Source: CAD feature listing. Evaluate the final solid. Frame: model axes, mm. Face numbers are marked on the shaded views. A direction names the side the tool comes from. Round coordinates to 2 decimals unless told otherwise and drop trailing zeros. Write each loop counter-clockwise with the first axis right and the second up, starting at its lowest first coordinate (ties: lowest second). Pieces come first, ordered by that corner, then holes. Notation, with made-up numbers: (87, 72.5) -> (120, 72.5) arc R19 cw to (120, 105.5) -> close; hole circle Ø5 at (-31.75, -33). An arc over 180 degrees is marked (long way). Return JSON: item names as keys, results as strings. Group by question number.
from build123d import *

# Parameters (mm, degrees)
SKETCH1_R             = 10.728678925
BOSS_EXTRUDE1_DEPTH   = 25.4
BOSS_EXTRUDE1_2_DEPTH = 25.4
SKETCH2_W             = 21.45735785
SKETCH2_H             = 6.35
BOSS_EXTRUDE2_DEPTH   = 17.0688


with BuildPart() as part:
    # Sketch1 → Boss-Extrude1 (new body)
    with BuildSketch(Plane.XY):
        Circle(SKETCH1_R)
    extrude(amount=BOSS_EXTRUDE1_DEPTH)



with BuildPart() as body_2:
    # Sketch1 → Boss-Extrude1 2 (new body)
    with BuildSketch(Plane.XY):
        Polygon((-35.51174, 17.0688), (35.51174, 17.0688), (35.51174, 69.1134), (6.3246, 69.1134), (6.3246, 65.3034), (31.70428, 65.3034), (31.70428, 27.2288), (-31.70428, 27.2288), (-31.70428, 65.3034), (-6.3246, 65.3034), (-6.3246, 69.1134), (-35.51174, 69.1134), align=None)
    extrude(amount=BOSS_EXTRUDE1_2_DEPTH)


with BuildPart() as part_1:
    add(part.part)

    add(body_2.part)  # Boss-Extrude2 merges body 2
    # Sketch2 → Boss-Extrude2 (add)
    with BuildSketch(Plane.XZ.offset(-17.0688)):
        with Locations((0, 3.175)):
            Rectangle(SKETCH2_W, SKETCH2_H)
    extrude(amount=BOSS_EXTRUDE2_DEPTH)


solid = part_1.part
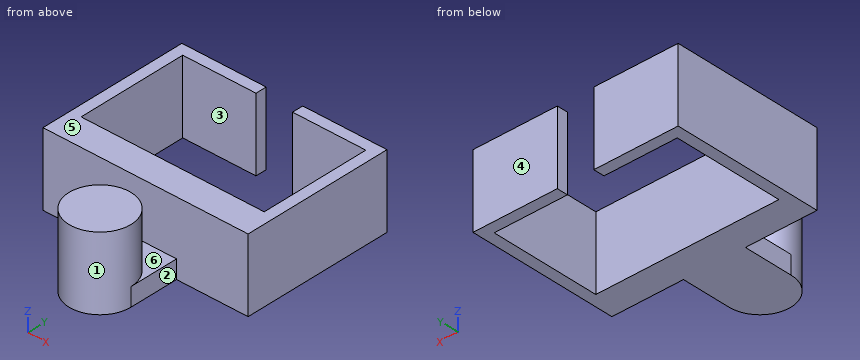
Item 1: First-contact query: pin 1 Ø4 at (y, z) = (-2, 15.5) entering from +X; pin 2 Ø5 at (x, z) = (15, 10) entering from -Y; pin 3 Ø7.5 at (x, z) = (-9.5, 11.5) entering from -Y. Flat tips, straight axial feed; report the tip coordinate or a pass-through.
Item 2: Cut plane A-A on y = 43. Output: boundary loops of the cut face in (x, z), and give its area (3 significant figures).
Item 3: Pull-direction query (Y, two-part tool) for the marked faces 4, 5 and 6; classes: +Y half, -Y half, draft (parallel to the pull), parting line (faces both ways), or undercut.
Item 4: Cut plane D-D on x = 0. Output: boundary loops of the cut face in (y, z), and give its area (3 significant figures).
Item 5: Cut plane B-B on z = 21. Output: boundary loops of the cut face in (x, y).
Item 6: Set-up query: the marked faces 1, 2 and 3. Return all of +Z, -Z, +X, -X, +Y, -Y with unobstructed straight access to the full face (end or side cutting, diameter ignored); none if empty.
Item 7: Cut plane C-C on x = -24. Output: boundary loops of the cut face in (y, z), and give its area (3 significant figures).
Item 8: Material intervals for probe 1 along Y at (x, z) = (-14, 18); probe 2 along Y at (x, z) = (-7.5, 13.5); probe 3 along X at (y, z) = (33, 7), sorted ascending.
Here are the results:
{
 "1": {"pin 1": "stops at x = 10.73", "pin 2": "stops at y = 17.07", "pin 3": "stops at y = -9.06"},
 "2": {"outline": "(-35.51, 0) -> (-31.7, 0) -> (-31.7, 25.4) -> (-35.51, 25.4) -> close; (31.7, 0) -> (35.51, 0) -> (35.51, 25.4) -> (31.7, 25.4) -> close", "area": "193 mm^2"},
 "3": {"face 4": "+Y half", "face 5": "draft", "face 6": "undercut"},
 "4": {"outline": "(-10.73, 0) -> (27.23, 0) -> (27.23, 25.4) -> (17.07, 25.4) -> (17.07, 6.35) -> (10.73, 6.35) -> (10.73, 25.4) -> (-10.73, 25.4) -> close", "area": "843 mm^2"},
 "5": {"outline": "(-35.51, 17.07) -> (35.51, 17.07) -> (35.51, 69.11) -> (6.32, 69.11) -> (6.32, 65.3) -> (31.7, 65.3) -> (31.7, 27.23) -> (-31.7, 27.23) -> (-31.7, 65.3) -> (-6.32, 65.3) -> (-6.32, 69.11) -> (-35.51, 69.11) -> close; circle Ø21.46 at (0, 0)"},
 "6": {"face 1": "+Z", "face 2": "+Z, -Z, +X, -Y", "face 3": "+Z, -Z"},
 "7": {"outline": "(17.07, 0) -> (27.23, 0) -> (27.23, 25.4) -> (17.07, 25.4) -> close; (65.3, 0) -> (69.11, 0) -> (69.11, 25.4) -> (65.3, 25.4) -> close", "area": "355 mm^2"},
 "8": {"probe 1": "y = 17.07 to 27.23, 65.3 to 69.11", "probe 2": "y = -7.67 to 7.67, 17.07 to 27.23, 65.3 to 69.11", "probe 3": "x = -35.51 to -31.7, 31.7 to 35.51"}
}
